Autodesk Fusion 360 part; units mm, degrees
sketch "スケッチ1" plane through (0, 0, 0) normal (0, 0, 1) x (1, 0, 0)
  line L0 (-21.5, 91) -> (-68.5, 91)
  line L1 (-68.5, 91) -> (-68.5, -91)
  line L2 (-68.5, -91) -> (-21.5, -91)
  line L3 (68.5, -30) -> (68.5, 80)
  line L4 (60.2198, 80) -> (-68.5, -91) construction
  line L5 (-68.5, 91) -> (45.5182, -60.4695) construction
  line L6 (-21.5, 91) -> (-21.5, 80)
  line L7 (-21.5, 80) -> (68.5, 80)
  line L8 (-68.5, -91) -> (-21.5, -91) construction
  line L9 (68.5, -50) -> (-21.5, -91)
  line L10 (68.5, -50) -> (-21.5, -50)
  line L11 (-21.5, -50) -> (-21.5, -30)
  line L12 (-21.5, -30) -> (68.5, -30)
  dimension "d2" = 182
  dimension "d5" = 47
  dimension "d7" = 90
  dimension "d8" = 20
extrude "押し出し1" add sketch "スケッチ1" along normal blind 6
chamfer "面取り1" distance 15 angle 45 2 edges at (-68.5, -91, 3) (-68.5, 91, 3)
sketch "スケッチ2" plane through (0, 0, 6) normal (0, 0, 1) x (-1, 0, 0)
  line L0 (53.5, -91) -> (68.5, -76)
  line L1 (68.5, -76) -> (68.5, 76)
  line L2 (68.5, 76) -> (53.5, 91)
  line L3 (53.5, 91) -> (21.5, 91)
  line L4 (21.5, 91) -> (-68.5, 50)
  line L5 (-68.5, 50) -> (21.5, 50)
  line L6 (21.5, 50) -> (21.5, 30)
  line L7 (21.5, 30) -> (-68.5, 30)
  line L8 (-68.5, 30) -> (-68.5, -80)
  line L9 (-68.5, -80) -> (21.5, -80)
  line L10 (21.5, -80) -> (21.5, -91)
  line L11 (21.5, -91) -> (53.5, -91)
  line L12 (-68.5, -80) -> (-28.5, -80) construction
  line L13 (-28.5, -80) -> (-28.5, -50) construction
  line L14 (-28.5, -50) -> (-68.5, -50) construction
  line L15 (-68.5, -50) -> (-68.5, -80) construction
  line L16 (-28.5, -50) -> (-28.5, 0) construction
  point P0 (-28.5, -50)
  point P1 (-28.5, 0)
  dimension "d12" = 40
  dimension "d13" = 30
  dimension "d14" = 50
hole "穴1" at (28.5, 0, 6) at (28.5, 50, 6) direction (0, 0, -1) diameter 18 end through all
equation "d5 = 15 mm + 32 mm"
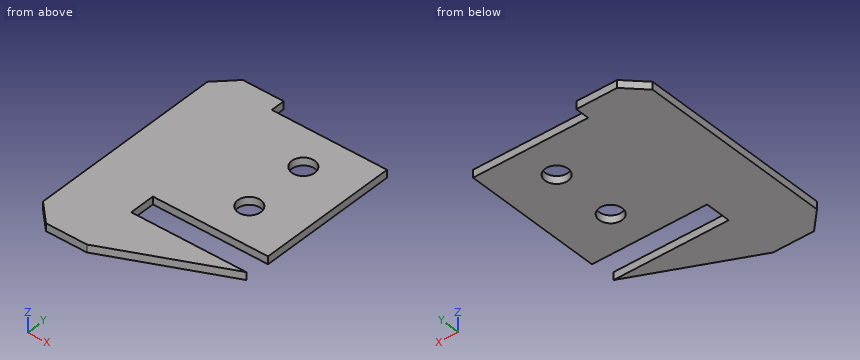
Geometry: final body of the model. Coordinates: model frame, mm. Give positions to 0.01 mm unless a question says otherwise; leave off trailing zeros. Loops run counter-clockwise (first coordinate to the right, second up) from the corner with the lowest first, then second, coordinate; pieces in that order, holes last. Notation, with made-up numbers: M -39,60 L -13,60 A24 ccw -13,75 Z; hole C -2,85 d2. An arc over 180 degrees is marked long. Put each result on its own line as item: value. Start each with the question number.
1) Cut plane A-A (y = 0). Output: boundary loops of the cut face in (x, z).
2) Cut plane B-B (z = 4.45). Output: boundary loops of the cut face in (x, y), then the cut area to 3 significant figures.
3) Ray query, line 1 along X through (y, z) = (0, 4.5); line 2 along Y through (x, z) = (28.5, 1.6); line 3 along Y through (x, z) = (28, 3.5). Return the intervals inside material, ascending.
4) Cut plane C-C (x = 21.5). Output: boundary loops of the cut face in (y, z), then the cut area to 3 significant figures.
5) Contact query for flat-ended pins moving along their axis: pin 1 (2 mm diameter, centred on x = 34, z = 1.5, fed in from +Y); pin 2 (3 mm diameter, centred on y = 86, z = 3, fed in from +X); pin 3 (4 mm diameter, centred on x = -47.5, y = 43, fed in from -Z); pin 4 (1 mm diameter, centred on x = -17, z = 5.5, fed in from -Y). Output: stop coordinate, or through.
6) Cut plane D-D (x = -13). Output: boundary loops of the cut face in (y, z).
Verdict:
1. outline: M -68.5,0 L 19.5,0 L 19.5,6 L -68.5,6 Z; M 37.5,0 L 68.5,0 L 68.5,6 L 37.5,6 Z
2. outline: M -68.5,-76 L -53.5,-91 L -21.5,-91 L 68.5,-50 L -21.5,-50 L -21.5,-30 L 68.5,-30 L 68.5,80 L -21.5,80 L -21.5,91 L -53.5,91 L -68.5,76 Z; hole C 28.5,0 d18; hole C 28.5,50 d18
2. area: 19,600 mm2
3. line 1: -68.5 to 19.5, 37.5 to 68.5
3. line 2: -68.22 to -50, -30 to -9, 9 to 41, 59 to 80
3. line 3: -68.45 to -50, -30 to -8.99, 8.99 to 41.01, 58.99 to 80
4. outline: M -71.41,0 L -50,0 L -50,6 L -71.41,6 Z; M -30,0 L -5.66,0 L -5.66,6 L -30,6 Z; M 5.66,0 L 44.34,0 L 44.34,6 L 5.66,6 Z; M 55.66,0 L 80,0 L 80,6 L 55.66,6 Z
4. area: 653 mm2
5. pin 1: y = 80
5. pin 2: x = -21.5
5. pin 3: z = 0
5. pin 4: y = -89.18
6. outline: M -87.13,0 L -50,0 L -50,6 L -87.13,6 Z; M -30,0 L 80,0 L 80,6 L -30,6 Z
